Design review of the part built by this model. Coordinates are the model's own, in mm. A direction names the side the tool comes from. Coordinates: 2 decimals unless noted, no trailing zeros. Order: outer loops, then holes, each group sorted by start corner. A loop starts at its lowest first (then second) coordinate and runs counter-clockwise, first axis right, second up. Notation, with made-up numbers: (7, 31.5) - (51, 31.5) arc R13 cw to (51, 55.5) - close; hole circle Ø10 at (78, 34). An arc over 180 degrees is marked (long way). Write each question's results on one line, items separated by ' | '. Start each with the question number.
```python
from build123d import *

# Parameters (mm, degrees)
SKETCH1_W           = 27.22
SKETCH1_H           = 50.8
BOSS_EXTRUDE1_DEPTH = 7.62
SKETCH2_R           = 2.05
CUT_EXTRUDE1_DEPTH  = 7.62
SKETCH3_R           = 3.3782
CUT_EXTRUDE2_DEPTH  = 2.54
SKETCH4_W           = 27.22
SKETCH4_H           = 19.05
BOSS_EXTRUDE2_DEPTH = 25.4
SKETCH5_W           = 27.22
SKETCH5_H           = 33.02
BOSS_EXTRUDE3_DEPTH = 25.4
SKETCH7_W           = 27.22
SKETCH7_H           = 6.35
CUT_EXTRUDE3_DEPTH  = 38.1
CUT_EXTRUDE4_DEPTH  = 27.94
CUT_EXTRUDE5_DEPTH  = 27.94
CUT_EXTRUDE6_DEPTH  = 27.94
SKETCH12_W          = 27.22
SKETCH12_H          = 5.08
BOSS_EXTRUDE5_DEPTH = 20.32
CUT_EXTRUDE8_DEPTH  = 12.7
SKETCH16_R          = 4.826
CUT_EXTRUDE9_DEPTH  = 2.54


with BuildPart() as part:
    # Sketch1 → Boss-Extrude1 (new body)
    with BuildSketch(Plane(origin=(0, 0, 0), x_dir=(1, 0, 0), z_dir=(0, 1, 0))):
        with Locations((-0.346834532, 16.982733813)):
            Rectangle(SKETCH1_W, SKETCH1_H)
    extrude(amount=BOSS_EXTRUDE1_DEPTH)

    # Sketch2 → Cut-Extrude1 (cut)
    with BuildSketch(Plane(origin=(0, 7.62, 0), x_dir=(1, 0, 0), z_dir=(0, 1, 0))):
        with Locations(Location((-9.346834532, 8.232733813, 0), (0, 0, 270))):
            Circle(SKETCH2_R)
    cut_extrude1 = extrude(amount=-CUT_EXTRUDE1_DEPTH, mode=Mode.SUBTRACT)

    # Sketch3 → Cut-Extrude2 (cut)
    with BuildSketch(Plane(origin=(0, 7.62, 0), x_dir=(1, 0, 0), z_dir=(0, 1, 0))):
        with Locations(Location((-9.346834532, 8.232733813, 0), (0, 0, 270))):
            Circle(SKETCH3_R)
    cut_extrude2 = extrude(amount=-CUT_EXTRUDE2_DEPTH, mode=Mode.SUBTRACT)

    # Mirror1: Cut-Extrude1, Cut-Extrude2 across plane
    add(cut_extrude1.mirror(Plane.ZY.offset(0.346834532)), mode=Mode.SUBTRACT)
    add(cut_extrude2.mirror(Plane.ZY.offset(0.346834532)), mode=Mode.SUBTRACT)

    # Sketch4 → Boss-Extrude2 (add)
    with BuildSketch(Plane(origin=(0, 7.62, 0), x_dir=(1, 0, 0), z_dir=(0, 1, 0))):
        with Locations((-0.346834532, 32.857733813)):
            Rectangle(SKETCH4_W, SKETCH4_H)
    extrude(amount=BOSS_EXTRUDE2_DEPTH)

    # Sketch5 → Boss-Extrude3 (add)
    with BuildSketch(Plane(origin=(0, 0, -42.382733813), x_dir=(-1, 0, 0), z_dir=(0, 0, -1))):
        with Locations((0.346834532, 16.51)):
            Rectangle(SKETCH5_W, SKETCH5_H)
    extrude(amount=BOSS_EXTRUDE3_DEPTH)

    # Sketch7 → Cut-Extrude3 (cut)
    with BuildSketch(Plane(origin=(0, 0, -67.782733813), x_dir=(-1, 0, 0), z_dir=(0, 0, -1))):
        with Locations((0.346834532, 3.175)):
            Rectangle(SKETCH7_W, SKETCH7_H)
    extrude(amount=-CUT_EXTRUDE3_DEPTH, mode=Mode.SUBTRACT)

    # Sketch8 → Cut-Extrude4 (cut)
    with BuildSketch(Plane.ZY.offset(13.956834532)):
        Polygon((-29.682733813, 6.35), (-29.682733813, 25.4), (-55.082733813, 6.35), align=None)
    extrude(amount=-CUT_EXTRUDE4_DEPTH, mode=Mode.SUBTRACT)

    # Sketch9 → Cut-Extrude5 (cut)
    with BuildSketch(Plane.ZY.offset(13.956834532)):
        Polygon((-67.782733813, 33.02), (-67.782733813, 6.35), (-29.682733813, 33.02), align=None)
    extrude(amount=-CUT_EXTRUDE5_DEPTH, mode=Mode.SUBTRACT)

    # Sketch11 → Cut-Extrude6 (cut)
    with BuildSketch(Plane.ZY.offset(13.956834532)):
        Polygon((-61.432733813, 6.35), (-61.432733813, 10.795), (-67.782733813, 6.35), align=None)
    extrude(amount=-CUT_EXTRUDE6_DEPTH, mode=Mode.SUBTRACT)

    # Sketch12 → Boss-Extrude5 (add)
    with BuildSketch(Plane(origin=(0, 36.105982328, -25.27418763), x_dir=(1, 0, 0), z_dir=(0, 0.8192319205190405, -0.5734623443633285))):
        with Locations((-0.346834532, 41.597130497)):
            Rectangle(SKETCH12_W, SKETCH12_H)
    extrude(amount=BOSS_EXTRUDE5_DEPTH)

    # Sketch15 → Cut-Extrude8 (cut)
    with BuildSketch(Plane(origin=(0, 36.105982328, -25.27418763), x_dir=(1, 0, 0), z_dir=(0, 0.8192319205190405, -0.5734623443633285))):
        with BuildLine():
            ThreePointArc((2.955165468, 28.897130497), (1.988032059, 31.231997088), (-0.346834532, 32.199130497))
            Line((-0.346834532, 32.199130497), (-0.346834532, 25.595130497))
            ThreePointArc((-0.346834532, 25.595130497), (1.988032059, 26.562263905), (2.955165468, 28.897130497))
        make_face()
        with BuildLine():
            Line((-0.346834532, 25.595130497), (-0.346834532, 32.199130497))
            ThreePointArc((-0.346834532, 32.199130497), (-3.648834532, 28.897130497), (-0.346834532, 25.595130497))
        make_face()
    extrude(amount=-CUT_EXTRUDE8_DEPTH, mode=Mode.SUBTRACT)

    # Sketch16 → Cut-Extrude9 (cut)
    with BuildSketch(Plane(origin=(0, 30.50371223, -22.877784173), x_dir=(1, 0, 0), z_dir=(0, -0.7999999999999999, 0.6000000000000003))):
        with Locations(Location((-0.346834532, -27.662506101, 0), (0, 0, 270))):
            Circle(SKETCH16_R)
    extrude(amount=-CUT_EXTRUDE9_DEPTH, mode=Mode.SUBTRACT)


solid = part.part
```
(1) Take a section at B-B (y = 22.5). State the section outline as (x, z) points, plus the area to 3 significant figures.
(2) Tool access review of faces 4 (the face through (-6.498, 6.368, -6.417)), 5 (the face through (0, 6.35, -58)), 6 (the face through (-1, 7.62, -8)): name each direction out of +Z, -Z, +X, -X, +Y, -Y from which nothing blocks a thin tool from reaching the whole face with its end or side.
(3) Take a section at D-D (z = -35.5). State the section outline as (x, y) points, plus the area to 3 significant figures.
(4) Take a section at C-C (y = 26.5). State the section outline as (x, z) points.
(5) Clearance check with flat-ended pins moving along their axes: pin 1 (8 mm diameter, centred on x = -7, z = -9, fed in from +Y); pin 2 (2 mm diameter, centred on x = 6, y = 8, fed in from -Z); pin 3 (5 mm diameter, centred on x = 7.5, z = -30, fed in from -Y); pin 4 (2 mm diameter, centred on y = 27.5, z = -39.5, fed in from +X). State where each tip first meets the part, or that it passes through.
(6) Mouldability with a two-part tool opening along Y and no side actions: class faces 1 (the face through (7.268, 2.576, -9.744)), 2 (the face through (-2.42, 14.05, -49.05)), 3 (the face through (11, 5.08, -8)) as +Y half, -Y half, draft (parallel to the pull), parting line (faces both ways), or undercut.
(7) To check wall thickness, follow line 1 along Z through (x, y) = (-9.5, 3); line 2 along Z through (x, y) = (2.5, 14); line 3 along Z through (x, y) = (8.25, 14). State the ranges of each line that lie inside material, in increasing order. Write a range as [from, to].
Worked out:
1) outline: (-13.96, -69.63) - (13.26, -69.63) - (13.26, -63.43) - (-13.96, -63.43) - close; (-13.96, -44.71) - (13.26, -44.71) - (13.26, -33.55) - (-13.96, -33.55) - close; (-13.96, -29.68) - (13.26, -29.68) - (13.26, -23.33) - (-13.96, -23.33) - close | area: 645 mm^2
2) face 4: +Y | face 5: -Z, +X, -X, -Y | face 6: +Z, +X, -X, +Y
3) outline: (-13.96, 21.04) - (13.26, 21.04) - (13.26, 28.95) - (-13.96, 28.95) - close | area: 215 mm^2
4) outline: (-13.96, -72.43) - (13.26, -72.43) - (13.26, -66.23) - (-13.96, -66.23) - close; (-13.96, -39) - (13.26, -39) - (13.26, -23.33) - (-13.96, -23.33) - close
5) pin 1: y = 7.62 | pin 2: z = -61.43 | pin 3: y = 0 | pin 4: through
6) face 1: draft | face 2: undercut | face 3: +Y half
7) line 1: [-29.68, -10.28], [-6.19, 8.42] | line 2: [-63.68, -57.48], [-56.85, -49.12], [-29.68, -23.33] | line 3: [-63.68, -57.48], [-56.85, -44.88], [-29.68, -23.33]
